Here's how the part is built. I have some questions about the finished solid (model axes, mm). Face numbers are marked on the shaded views. A direction names the side the tool comes from. Round coordinates to 2 decimals unless told otherwise and drop trailing zeros. Write each loop counter-clockwise with the first axis right and the second up, starting at its lowest first coordinate (ties: lowest second). Pieces come first, ordered by that corner, then holes. Notation, with made-up numbers: (85.5, 16) -> (129.5, 16) arc R23 cw to (129.5, 43) -> close; hole circle Ø11 at (-39.5, -25.5). An arc over 180 degrees is marked (long way). Answer in a Markdown table with one row per item.
Autodesk Inventor part; units mm, degrees
ref_plane "YZ Plane" through (0, 0, 0) normal (1, 0, 0) x (0, 1, 0)
ref_plane "XZ Plane" through (0, 0, 0) normal (0, 1, 0) x (-1, 0, 0)
ref_plane "XY Plane" through (0, 0, 0) normal (0, 0, 1) x (1, 0, 0)
sketch "Sketch1" plane through (0, 0, 0) normal (0, 1, 0) x (-1, 0, 0)
  line L0 (0, -12.7) -> (0, -25.4)
  line L1 (0, -25.4) -> (50.8, -25.4)
  line L2 (50.8, -25.4) -> (50.8, 0)
  line L3 (50.8, 0) -> (19.05, 0)
  line L4 (19.05, 0) -> (19.05, -12.7)
  line L5 (19.05, -12.7) -> (0, -12.7)
  point P0 (0, 0)
  dimension "d0" = 12.7
  dimension "d1" = 50.8
  dimension "d2" = 25.4
  dimension "d3" = 31.75
  dimension "d4" = 12.7
extrude "Extrusion1" add sketch "Sketch1" along normal blind 38.1
chamfer "Chamfer1" distance 19.05 distance2 38.1 1 edges at (-19.05, 38.1, -6.35) measured on face at (-40.2167, 38.1, -12.7)
chamfer "Chamfer2" distance 12.7 distance2 19.05 1 edges at (0, 38.1, -19.05) measured on face at (-23.2833, 38.1, -21.1667)
properties part number "7.1 Part 4"
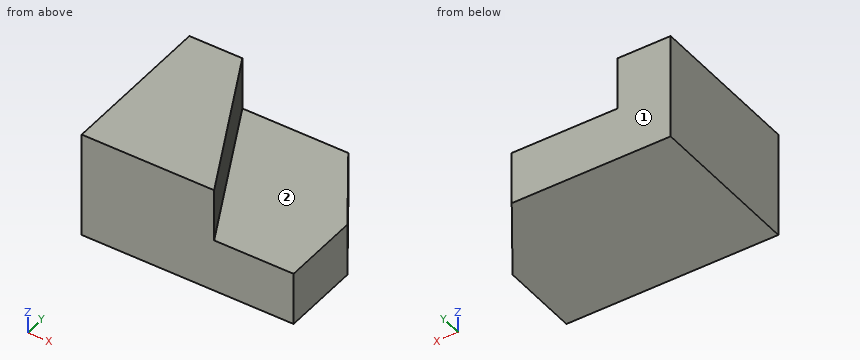
1) I want a section at A-A, the plane z = -22.5. List the corners of the cut face in (x, y) for me.
Response:
| item | result |
|---|---|
| outline | (-50.8, 0) -> (0, 0) -> (0, 19.05) -> (-12.7, 38.1) -> (-50.8, 38.1) -> close |
2) I want a section at B-B, the plane x = -14.5. List the corners of the cut face in (y, z) for me, and give its area (3 significant figures).
Response:
| item | result |
|---|---|
| outline | (0, -25.4) -> (38.1, -25.4) -> (38.1, -12.7) -> (0, -12.7) -> close |
| area | 484 mm^2 |
3) I want a section at C-C, the plane y = 17. List the corners of the cut face in (x, z) for me, and give its area (3 significant figures).
Response:
| item | result |
|---|---|
| outline | (-50.8, -25.4) -> (0, -25.4) -> (0, -12.7) -> (-27.55, -12.7) -> (-27.55, 0) -> (-50.8, 0) -> close |
| area | 940 mm^2 |
4) For pin 1 (1.5 mm diameter, centred on y = 33, z = -7, fed in from +X); pin 2 (4 mm diameter, centred on x = -22, y = 23, fed in from +Z), each with a flat end and sliding along its axis, tell me the tip position at first contact or that it passes through.
Response:
| item | result |
|---|---|
| pin 1 | stops at x = -35.17 |
| pin 2 | stops at z = -12.7 |
5) I need wall thicknesses on line 1 (Z direction, x = -29, y = 20); line 2 (X direction, y = 30.5, z = -2); line 3 (X direction, y = 27, z = -16.75). Which ranges of each line are inside material? Lowest first, please. Write a range as [from, to].
Response:
| item | result |
|---|---|
| line 1 | z = [-25.4, -12.7] |
| line 2 | x = [-50.8, -34.3] |
| line 3 | x = [-50.8, -5.3] |
6) Which directions (+Z, -Z, +X, -X, +Y, -Y) give clear straight access to the entire face, cutting with the end or side of a thin tool? Please do the marked faces 1 and 2.
Response:
| item | result |
|---|---|
| face 1 | +Z, -Z, +X, -X, +Y |
| face 2 | +Z, +X, +Y |
